Can you work these out from the model? Positions are in its coordinate system, mm. Coordinates: 2 decimals unless noted, no trailing zeros. Write each loop counter-clockwise with the first axis right and the second up, starting at its lowest first coordinate (ties: lowest second). Pieces come first, ordered by that corner, then holes. Notation, with made-up numbers: (-0.75, 64.5) - (19.25, 64.5) arc R25 cw to (19.25, 103.5) - close; hole circle Ø4 at (76, 88.25). An arc over 180 degrees is marked (long way). Use one line per item in the form item = value. Start each with the question number.
(1) If we section it at C-C on z = -126: Please give me the cut outline in (x, y).
(2) If we section it at A-A on z = -83: Please give me the cut outline in (x, y), then the cut area to 3 significant figures.
(3) If we section it at D-D on y = 1.8: Give the number of separate pieces and of enclosed holes in the cut face, then the cut area to 3 significant figures.
(4) For pin 1 Ø2.5 at (y, z) = (3, 84.5) entering from +X; pin 2 Ø1.5 at (y, z) = (3, -91) entering from -X; pin 3 Ø1.5 at (y, z) = (2.5, -54) entering from -X, each with a flat end and sliding along its axis, tell me the tip position at first contact or that it passes through.
(5) If I drill on probe 1 along Z at (x, y) = (0, 3.4); probe 2 along X at (y, z) = (1.35, 2), over which ranges is the centre line in solid material (lowest first)? Write a range as from..to.
(6) If we section it at B-B on x = 93.5: Please give me the cut outline in (y, z).
Autodesk Fusion 360 part; units mm, degrees
sketch "Sketch1" plane through (0, 0, 0) normal (0, 1, 0) x (1, 0, 0)
  circle A0 centre (0, 0) radius 145
  circle A1 centre (0, 0) radius 140
  circle A2 centre (0, 0) radius 25
  circle A3 centre (0, 0) radius 30
  line L0 (-2.5, 140) -> (-2.5, 29.8957)
  line L1 (2.5, 140) -> (2.5, 29.8957)
  circle A4 centre (0, 0) radius 105
  circle A5 centre (0, 0) radius 100
  circle A6 centre (0, 0) radius 65
  circle A7 centre (0, 0) radius 60
  line L2 (-97.2272, 100.7627) -> (-19.3717, 22.9072)
  line L3 (-100.7627, 97.2272) -> (-22.9072, 19.3717)
  line L4 (-140, 2.5) -> (-29.8957, 2.5)
  line L5 (-140, -2.5) -> (-29.8957, -2.5)
  line L6 (-100.7627, -97.2272) -> (-22.9072, -19.3717)
  line L7 (-97.2272, -100.7627) -> (-19.3717, -22.9072)
  line L8 (-2.5, -140) -> (-2.5, -29.8957)
  line L9 (2.5, -140) -> (2.5, -29.8957)
  line L10 (97.2272, -100.7627) -> (19.3717, -22.9072)
  line L11 (100.7627, -97.2272) -> (22.9072, -19.3717)
  line L12 (140, -2.5) -> (29.8957, -2.5)
  line L13 (140, 2.5) -> (29.8957, 2.5)
  line L14 (100.7627, 97.2272) -> (22.9072, 19.3717)
  line L15 (97.2272, 100.7627) -> (19.3717, 22.9072)
  dimension "d1" = 290
  dimension "d2" = 280
  dimension "d3" = 50
  dimension "d4" = 60
  dimension "d7" = 210
  dimension "d8" = 130
  dimension "d10" = 360
extrude "Extrude1" add sketch "Sketch1" along normal blind 5 contours A0 | A1 A4 L12 L13 | A1 A4 L14 L15 | A4 A5 L13 L14 | A4 A5 L12 L13 | A1 A4 L10 L11 | A4 A5 L11 L12 | A4 A5 L14 L15 | A5 A6 L12 L13 | A4 A5 L10 L11 | A1 L0 L1 A4 | L1 A4 A5 L15 | A5 A6 L14 L15 | A6 A7 L13 L14 | A6 A7 L12 L13 | A1 A4 L8 L9 | A4 A5 L9 L10 | A5 A6 L10 L11 | A6 A7 L11 L12 | L0 L1 A4 A5 | A6 A7 L14 L15 | A3 A7 L12 L13 | A4 A5 L8 L9 | A6 A7 L10 L11 | A1 A4 L2 L3 | L0 A4 A5 L2 | L0 L1 A5 A6 | L1 A6 A7 L15 | A3 A7 L14 L15 | A3 | A1 A4 L6 L7 | A4 A5 L7 L8 | A5 A6 L8 L9 | A6 A7 L9 L10 | A3 A7 L10 L11 | A4 A5 L2 L3 | L0 L1 A6 A7 | A4 A5 L6 L7 | A6 A7 L8 L9 | A1 A4 L4 L5 | A4 A5 L3 L4 | A5 A6 L2 L3 | L0 A6 A7 L2 | A3 L0 L1 A7 | A4 A5 L5 L6 | A5 A6 L6 L7 | A6 A7 L7 L8 | A3 A7 L8 L9 | A4 A5 L4 L5 | A6 A7 L2 L3 | A6 A7 L6 L7 | A5 A6 L4 L5 | A6 A7 L3 L4 | A3 A7 L2 L3 | A6 A7 L5 L6 | A3 A7 L6 L7 | A6 A7 L4 L5 | A3 A7 L4 L5
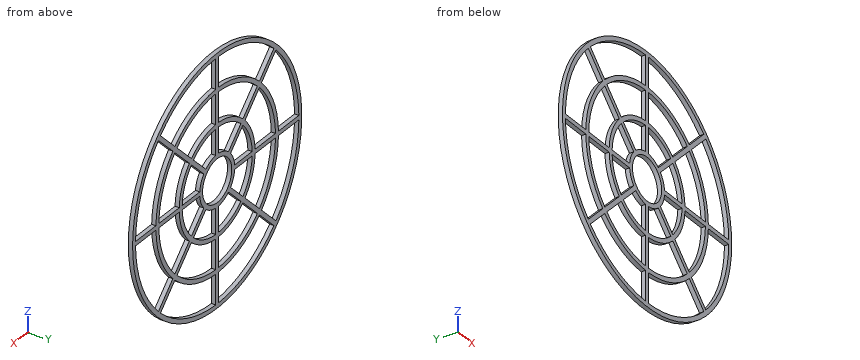
Reported:
q1.outline = (-71.76, 0) - (-61.02, 0) - (-61.02, 5) - (-71.76, 5) - close; (-2.5, 0) - (2.5, 0) - (2.5, 5) - (-2.5, 5) - close; (61.02, 0) - (71.76, 0) - (71.76, 5) - (61.02, 5) - close
q2.outline = (-118.89, 0) - (-112.74, 0) - (-112.74, 5) - (-118.89, 5) - close; (-86.54, 0) - (-79.46, 0) - (-79.46, 5) - (-86.54, 5) - close; (-64.31, 0) - (-55.78, 0) - (-55.78, 5) - (-64.31, 5) - close; (-2.5, 0) - (2.5, 0) - (2.5, 5) - (-2.5, 5) - close; (55.78, 0) - (64.31, 0) - (64.31, 5) - (55.78, 5) - close; (79.46, 0) - (86.54, 0) - (86.54, 5) - (79.46, 5) - close; (112.74, 0) - (118.89, 0) - (118.89, 5) - (112.74, 5) - close
q2.area = 243 mm2
q3.separate_pieces = 1
q3.enclosed_holes = 25
q3.area = 14,500 mm2
q4.pin_1 = 118.72
q4.pin_2 = -113.49
q4.pin_3 = -134.87
q5.probe_1 = -145..-25, 25..145
q5.probe_2 = -144.99..-24.92, 24.92..144.99
q6.outline = (0, -110.83) - (5, -110.83) - (5, -104.2) - (0, -104.2) - close; (0, -97.04) - (5, -97.04) - (5, -89.96) - (0, -89.96) - close; (0, -47.78) - (5, -47.78) - (5, -35.46) - (0, -35.46) - close; (0, -2.5) - (5, -2.5) - (5, 2.5) - (0, 2.5) - close; (0, 35.46) - (5, 35.46) - (5, 47.78) - (0, 47.78) - close; (0, 89.96) - (5, 89.96) - (5, 97.04) - (0, 97.04) - close; (0, 104.2) - (5, 104.2) - (5, 110.83) - (0, 110.83) - close
